Input: part model. Units: mm. Frame: model coordinates. A direction names the side the tool comes from. Round coordinates to 2 decimals unless told otherwise and drop trailing zeros. Order: outer loops, then holes, each group sorted by start corner. A loop starts at its lowest first (then second) coordinate and runs counter-clockwise, first axis right, second up. Notation, with made-up numbers: (37, 40.5) -> (45, 40.5) arc R15 ccw to (45, 51.5) -> close; hole circle Ø7 at (-7, -11.5). An arc over 180 degrees is marked (long way). Use a Markdown table: item, result.
from build123d import *

# Parameters (mm, degrees)
BOSS_EXTRUDE1_DEPTH      = 8.33
BOSS_EXTRUDE1_DEPTH_BACK = 8.33
SKETCH1_R                = 22.5
BOSS_EXTRUDE2_START      = 10
SKETCH2_R                = 7.5
BOSS_EXTRUDE2_DEPTH      = 20
SKETCH3_R                = 2.5
CUT_EXTRUDE2_DEPTH       = 10
BOSS_EXTRUDE3_DEPTH      = 25
BOSS_EXTRUDE3_DEPTH_BACK = 25
SKETCH7_R                = 5


with BuildPart() as part:
    # Sketch1 → Boss-Extrude1 (new, two sides: drawn at the far end of the back side and taken through both)
    with BuildSketch(Plane.XY.offset(-BOSS_EXTRUDE1_DEPTH_BACK)):
        Circle(SKETCH1_R)
    extrude(amount=BOSS_EXTRUDE1_DEPTH + BOSS_EXTRUDE1_DEPTH_BACK)

    # Sketch2 → Boss-Extrude2 (add)
    with BuildSketch(Plane(origin=(0, 0, 0), x_dir=(0, 0, -1), z_dir=(1, 0, 0)).offset(BOSS_EXTRUDE2_START)):
        Circle(SKETCH2_R)
    extrude(amount=BOSS_EXTRUDE2_DEPTH)

    # Sketch3 → Cut-Extrude2 (cut)
    with BuildSketch(Plane(origin=(30, 0, 0), x_dir=(0, 0, -1), z_dir=(1, 0, 0))):
        Circle(SKETCH3_R)
    extrude(amount=-CUT_EXTRUDE2_DEPTH, mode=Mode.SUBTRACT)

    # Sketch7 → Boss-Extrude3 (add, two sides: drawn at the far end of the back side and taken through both)
    with BuildSketch(Plane.XY.offset(-BOSS_EXTRUDE3_DEPTH_BACK)):
        Circle(SKETCH7_R)
    extrude(amount=BOSS_EXTRUDE3_DEPTH + BOSS_EXTRUDE3_DEPTH_BACK)


solid = part.part
1) Cut plane C-C on y = 0. Return loops of the section in (x, z), and give its area (3 significant figures).
Results found:
| item | result |
|---|---|
| outline | (-22.5, -8.33) -> (-5, -8.33) -> (-5, -25) -> (5, -25) -> (5, -8.33) -> (22.5, -8.33) -> (22.5, -7.5) -> (30, -7.5) -> (30, -2.5) -> (20, -2.5) -> (20, 2.5) -> (30, 2.5) -> (30, 7.5) -> (22.5, 7.5) -> (22.5, 8.33) -> (5, 8.33) -> (5, 25) -> (-5, 25) -> (-5, 8.33) -> (-22.5, 8.33) -> close |
| area | 1,150 mm² |
2) Cut plane A-A on z = 0. Return loops of the section in (x, y), and give its area (3 significant figures).
Results found:
| item | result |
|---|---|
| outline | (20, -2.5) -> (20, 2.5) -> (30, 2.5) -> (30, 7.5) -> (21.21, 7.5) arc R22.5 ccw (long way) to (21.21, -7.5) -> (30, -7.5) -> (30, -2.5) -> close |
| area | 1,660 mm² |
3) Cut plane D-D on z = 22.5. Return loops of the section in (x, y).
Results found:
| item | result |
|---|---|
| outline | circle Ø10 at (0, 0) |
4) Pull-direction query (Y, two-part tool) for faces 5 (the flat face through (30, 2, 2)), 6 (the cylindrical face through (25.545, 2.253, -7.154)), 7 (the cylindrical face through (25.07, -2.44, 0.54)); classes: +Y half, -Y half, draft (parallel to the pull), parting line (faces both ways), or undercut.
Results found:
| item | result |
|---|---|
| face 5 | draft |
| face 6 | parting line |
| face 7 | undercut |
5) Set-up query: faces 1 (the flat face through (20, 0, 0)), 2 (the cylindrical face through (-1.08, -4.88, 16.55)), 3 (the cylindrical face through (-1.08, -4.88, -16.78)), 4 (the flat face through (0, 0, 25)). Return all of +Z, -Z, +X, -X, +Y, -Y with unobstructed straight access to the full face (end or side cutting, diameter ignored); none if empty.
Results found:
| item | result |
|---|---|
| face 1 | +X |
| face 2 | +Z |
| face 3 | -Z |
| face 4 | +Z, +X, -X, +Y, -Y |
6) Cut plane B-B on x = 0. Return loops of the section in (y, z).
Results found:
| item | result |
|---|---|
| outline | (-22.5, -8.33) -> (-5, -8.33) -> (-5, -25) -> (5, -25) -> (5, -8.33) -> (22.5, -8.33) -> (22.5, 8.33) -> (5, 8.33) -> (5, 25) -> (-5, 25) -> (-5, 8.33) -> (-22.5, 8.33) -> close |
7) Pin query (flat end, axial travel): pin 1 Ø1 at (x, z) = (-15.5, 7) entering from -Y; pin 2 Ø10 at (x, z) = (1.5, 3.5) entering from -Y; pin 3 Ø4 at (x, z) = (20.5, -11) entering from -Y; pin 4 Ø12 at (x, z) = (18, -13) entering from +Y. Return the tip coordinate at first contact, or that it passes through.
Results found:
| item | result |
|---|---|
| pin 1 | stops at y = -16.77 |
| pin 2 | stops at y = -22.5 |
| pin 3 | passes through |
| pin 4 | stops at y = 17.43 |
8) Line query: L1, parallel to Y at x = 25.25, z = 0; L2, parallel to Z at x = 2.5, y = -7.5; L3, parallel to X at y = -3, z = 14. Output: solid intervals per line, ascending. Write a range as [from, to].
Results found:
| item | result |
|---|---|
| L1 | y = [-7.5, -2.5], [2.5, 7.5] |
| L2 | z = [-8.33, 8.33] |
| L3 | x = [-4, 4] |
